```python
from build123d import *

# Parameters (mm, degrees)
F2_R     = 18.3396458196
F2_R_2   = 12.8738649412
F3_DEPTH = 12.5
F4_COUNT = 4
F4_ANGLE = 270


with BuildPart() as f1:
    # F0 (on Front) → F1 (revolve)
    with BuildSketch(Plane.XZ):
        with BuildLine():
            ThreePointArc((59.3, -19.7423402868), (36.5537531047, -50.6958887284), (0, -62.5))
            Line((0, -62.5), (0, -82.5))
            ThreePointArc((0, -82.5), (58.3363094479, -58.3363094479), (82.5, 0))
            ThreePointArc((82.5, 0), (49.5385186032, 15.2315462117), (59.3, -19.7423402868))
        make_face()
    revolve(axis=Axis((0, 0, 14.3070674052), (0, 0, -1)))

    # F2 (on Front) → F3 (join, symmetric)
    with BuildSketch(Plane.XZ):
        with Locations((-82.6222896576, 0)):
            Circle(F2_R)
        with Locations((-82.6222896576, 0)):
            Circle(F2_R_2, mode=Mode.SUBTRACT)
    extrude(amount=F3_DEPTH, both=True)

    # F4: F1 ×4 about axis
    f4_axis = Axis((0, 0, 14.3070674052), (0, 0, -1))


with BuildPart() as f1_1:
    add(f1.part)
    for i in range(1, F4_COUNT):
        add(f1.part.rotate(f4_axis, i * F4_ANGLE / (F4_COUNT - 1)))


solid = f1_1.part
```
Geometry: final body of the model. Coordinates: model frame, mm. Give positions to 0.01 mm unless a question says otherwise; leave off trailing zeros. Loops run counter-clockwise (first coordinate to the right, second up) from the corner with the lowest first, then second, coordinate; pieces in that order, holes last. Notation, with made-up numbers: (-3, 61.25) -> (51, 61.25) arc R20 cw to (51, 69.25) -> close; hole circle Ø7 at (23, 28). An arc over 180 degrees is marked (long way). Return JSON: item names as keys, results as strings.
Item 1: Pin query (flat end, axial travel): P1, Ø20.5, axis at x = 82.62, z = 0, coming from the -Y side; P2, Ø13.5, axis at y = 93, z = 8.5, coming from the -X side; P3, Ø10, axis at x = 15.5, y = 4, coming from the -Z side; P4, Ø12, axis at x = 7.5, y = -56, coming from the +Z side. Return the tip coordinate at first contact, or that it passes through.
Filled in:
{"P1": "y = -39.61", "P2": "x = -12.5", "P3": "z = -81.76", "P4": "z = 20"}
Item 2: Section A-A, the plane z = -25.5. Output: boundary loops of the cut face in (x, y).
Filled in:
{"outline": "circle Ø156.92 at (0, 0); hole circle Ø114.12 at (0, 0)"}
Item 3: Section B-B, the plane z = -71. Output: boundary loops of the cut face in (x, y).
Filled in:
{"outline": "circle Ø84.03 at (0, 0)"}
Item 4: Line query: line 1 (Y direction, x = 16, z = -32.5); line 2 (Y direction, x = -2, z = -2.5); line 3 (Y direction, x = 27.5, z = 5). Output: solid intervals per line, ascending.
Filled in:
{"line 1": "-74.12 to -50.93, 50.93 to 74.12", "line 2": "-100.79 to -95.25, -82.44 to -42.61, 42.61 to 82.44, 95.25 to 100.79", "line 3": "-77.11 to -33.23, 33.23 to 77.11"}
Item 5: Mould query, pull axis X, two halves, no side actions, for faces 1 (the cylindrical face through (95.36, -0.17, 1.86)), 2 (the flat face through (-12.5, -95.4, 2.8)), 3 (the flat face through (-95.4, 12.5, 2.8)), 4 (the cylindrical face through (-95.36, 0.17, 1.86)). Classes: released by +X, released by -X, zero draft, split by the parting line, or undercut.
Filled in:
{"face 1": "undercut", "face 2": "released by -X", "face 3": "zero draft", "face 4": "undercut"}
